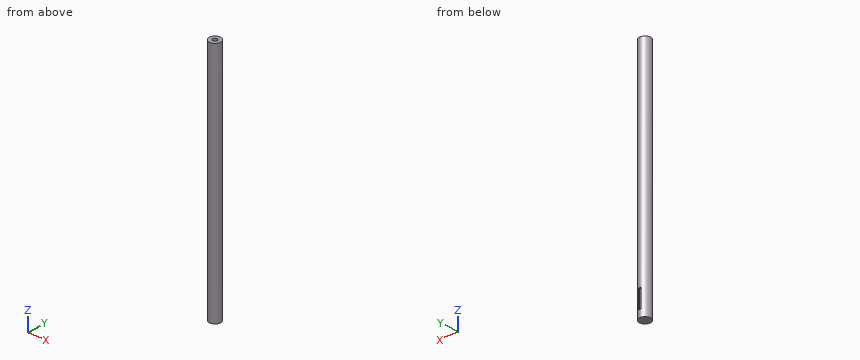
from build123d import *

# Parameters (mm, degrees)
SKETCH1_R           = 7.9375
EXTRUDE1_DEPTH      = 136.525
EXTRUDE1_DEPTH_BACK = 190.5
SKETCH2_R           = 3.175
CUT_EXTRUDE1_DEPTH  = 25.4
SKETCH3_W           = 25.4
SKETCH3_H           = 3.175
CUT_EXTRUDE2_DEPTH  = 1.5875


with BuildPart() as part:
    # Sketch1 → Extrude1 (new body, two sides)
    with BuildSketch(Plane.XY) as extrude1_sk:
        Circle(SKETCH1_R)
    extrude(amount=EXTRUDE1_DEPTH)
    extrude(extrude1_sk.sketch, amount=-EXTRUDE1_DEPTH_BACK)

    # Sketch2 → Cut-Extrude1 (cut)
    with BuildSketch(Plane.XY.offset(136.525)):
        Circle(SKETCH2_R)
    extrude(amount=-CUT_EXTRUDE1_DEPTH, mode=Mode.SUBTRACT)

    # Sketch3 → Cut-Extrude2 (cut, symmetric)
    with BuildSketch(Plane(origin=(0, 0, 0), x_dir=(0, 0, -1), z_dir=(1, 0, 0))):
        with Locations((168.275, 8.0264)):
            Rectangle(SKETCH3_W, SKETCH3_H)
    extrude(amount=CUT_EXTRUDE2_DEPTH, both=True, mode=Mode.SUBTRACT)


solid = part.part
Could you check a few things on this model? Use its own coordinates, in mm. Give positions to 0.01 mm unless a question says otherwise; leave off trailing zeros. Order: outer loops, then holes, each group sorted by start corner. A loop starts at its lowest first (then second) coordinate and runs counter-clockwise, first axis right, second up. Notation, with made-up numbers: (44, 25.5) - (86, 25.5) arc R23 cw to (86, 34.5) - close; hole circle Ø5 at (-13.75, 40). An arc over 180 degrees is marked (long way). Return JSON: item names as keys, results as strings. Group by question number.
Q1. Suppose I cut it at A-A, the plane y = 0. Please give me the cut outline in (x, z) (1 decimal).
Q2. Suppose I cut it at B-B, the plane z = -169.5. Please give me the cut outline in (x, y) (1 decimal).
Q3. Suppose I cut it at C-C, the plane z = -61. Please give me the cut outline in (x, y) (1 decimal).
Q4. Please list where these lines run through material, in increasing order: line 1 along Y through (x, z) = (0, 131.25) (1 decimal); line 2 along Z through (x, y) = (0.5, 7) (3 decimals); line 3 along Z through (x, y) = (-1.25, -1.5) (3 decimals). Write a range as [from, to].
Q5. Will these pins go through, and if not, where does the flat tip stop? pin 1 Ø6 at (x, z) = (-3.5, 26.5) entering from -Y; pin 2 Ø1.5 at (y, z) = (7, -173) entering from +X; pin 3 Ø6 at (y, z) = (5.5, 13.5) entering from +X.
Resolved:
{
 "1": {"outline": "(-7.9, -190.5) - (7.9, -190.5) - (7.9, 136.5) - (3.2, 136.5) - (3.2, 111.1) - (-3.2, 111.1) - (-3.2, 136.5) - (-7.9, 136.5) - close"},
 "2": {"outline": "(-1.6, 6.4) - (-1.6, 7.8) arc R7.9 ccw (long way) to (1.6, 7.8) - (1.6, 6.4) - close"},
 "3": {"outline": "circle Ø15.9 at (0, 0)"},
 "4": {"line 1": "y = [-7.9, -3.2], [3.2, 7.9]", "line 2": "z = [-190.5, -180.975], [-155.575, 136.525]", "line 3": "z = [-190.5, 111.125]"},
 "5": {"pin 1": "stops at y = -7.92", "pin 2": "stops at x = 4.89", "pin 3": "stops at x = 7.53"}
}
